The model under review builds one solid part; all positions refer to its coordinate system, in mm. Face numbers are marked on the shaded views. A direction names the side the tool comes from. Give positions to 0.01 mm unless a question says otherwise; leave off trailing zeros. Order: outer loops, then holes, each group sorted by start corner. A loop starts at its lowest first (then second) coordinate and runs counter-clockwise, first axis right, second up. Notation, with made-up numbers: (-13.5, 21.5) - (3.5, 21.5) arc R22 cw to (3.5, 55.5) - close; hole circle Ø9 at (7.25, 76). An arc over 180 degrees is marked (long way). Answer as CSV lines item,"result". Start each with the question number.
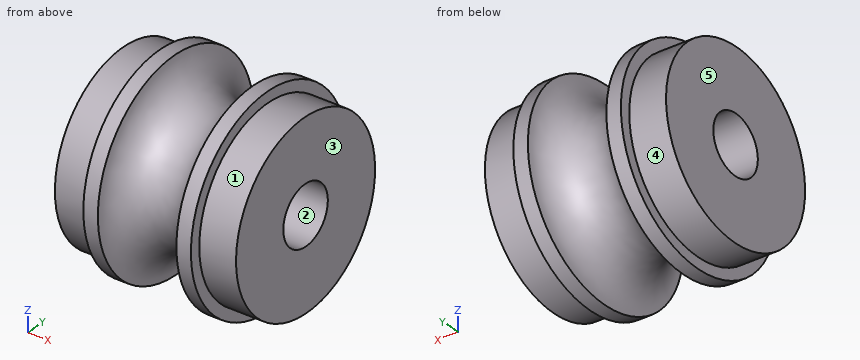
from build123d import *

# Parameters (mm, degrees)
SKETCH1_W           = 1.27
SKETCH1_H           = 8.89
SKETCH2_R           = 7.9375
BOSS_EXTRUDE1_DEPTH = 3.2131
BOSS_EXTRUDE2_START = 3.2131
SKETCH3_R           = 7.9375
BOSS_EXTRUDE2_DEPTH = 3.2131
SKETCH4_R           = 2.54
CUT_EXTRUDE1_DEPTH  = 21.210628532


with BuildPart() as part:
    # Sketch1 → Revolve1 (revolve)
    with BuildSketch(Plane.XY, mode=Mode.PRIVATE) as revolve1_sk:
        with BuildLine():
            ThreePointArc((0, 8.89), (3.429, 5.461), (6.858, 8.89))
            Line((6.858, 8.89), (6.858, 0))
            Line((6.858, 0), (0, 0))
            Line((0, 0), (0, 8.89))
        make_face()
        with Locations((-0.635, 4.445)):
            Rectangle(SKETCH1_W, SKETCH1_H)
        with Locations((7.493, 4.445)):
            Rectangle(SKETCH1_W, SKETCH1_H)
    revolve(revolve1_sk.sketch.rotate(Axis((0, 0, 0), (1, 0, 0)), 90), axis=Axis((0, 0, 0), (1, 0, 0)))

    # Sketch2 → Boss-Extrude1 (add)
    with BuildSketch(Plane(origin=(8.128, 0, 0), x_dir=(0, 0, -1), z_dir=(1, 0, 0))):
        Circle(SKETCH2_R)
    extrude(amount=BOSS_EXTRUDE1_DEPTH)

    # Sketch3 → Boss-Extrude2 (add)
    with BuildSketch(Plane.ZY.offset(1.27).offset(BOSS_EXTRUDE2_START)):
        with Locations(Location((0, 0, 0), (0, 0, 180))):
            Circle(SKETCH3_R)
    extrude(amount=-BOSS_EXTRUDE2_DEPTH)

    # Sketch4 → Cut-Extrude1 (cut, through all)
    with BuildSketch(Plane.ZY.offset(4.4831)):
        Circle(SKETCH4_R)
    extrude(amount=-CUT_EXTRUDE1_DEPTH, mode=Mode.SUBTRACT)


solid = part.part
Item 1: Take a section at D-D on x = 10. Write out the cut boundary in (y, z) (1 decimal), and give its area (3 significant figures).
Item 2: Take a section at A-A on y = 0. Write out the cut boundary in (x, z), and give its area (3 significant figures).
Item 3: Take a section at C-C on x = 7.25. Write out the cut boundary in (y, z), and give its area (3 significant figures).
Item 4: For line 1 along Z through (x, y) = (8.5, 1.75); line 2 along X through (y, z) = (6.75, 1); line 3 along X through (y, z) = (-3.75, 5.25), list the stretches that pass through material, from the lowest coordinate up.
Item 5: Clearance check with flat-ended pins moving along their axes: pin 1 (6 mm diameter, centred on x = 8, z = -5.5, fed in from -Y); pin 2 (1.5 mm diameter, centred on x = 4.5, z = -6.5, fed in from -Y). State where each tip first meets the part, or that it passes through.
Item 6: Machinability: for the marked faces 4 and 5, which of the approach directions +Z, -Z, +X, -X, +Y, -Y give a long, thin tool a straight path to every point of the face, cutting with its end or side? Answer none if there is none.
Item 7: Mouldability with a two-part tool opening along Z and no side actions: class the marked faces 1, 2 and 3 as released by +Z, released by -Z, zero draft, split by the parting line, or undercut.
Data:
1,outline,"circle Ø15.9 at (0, 0); hole circle Ø5.1 at (0, 0)"
1,area,"178 mm^2"
2,outline,"(-4.48, -7.94) - (-1.27, -7.94) - (-1.27, -8.89) - (0, -8.89) arc R3.43 cw to (6.86, -8.89) - (8.13, -8.89) - (8.13, -7.94) - (11.34, -7.94) - (11.34, -2.54) - (-4.48, -2.54) - close; (-4.48, 2.54) - (11.34, 2.54) - (11.34, 7.94) - (8.13, 7.94) - (8.13, 8.89) - (6.86, 8.89) arc R3.43 cw to (0, 8.89) - (-1.27, 8.89) - (-1.27, 7.94) - (-4.48, 7.94) - close"
2,area,"152 mm^2"
3,outline,"circle Ø17.78 at (0, 0); hole circle Ø5.08 at (0, 0)"
3,area,"228 mm^2"
4,line 1,"z = -7.74 to -1.84, 1.84 to 7.74"
4,line 2,"x = -4.48 to 0.69, 6.17 to 11.34"
4,line 3,"x = -4.48 to 1.02, 5.84 to 11.34"
5,pin 1,"stops at y = -8.53"
5,pin 2,"passes through"
6,face 4,"-X"
6,face 5,"+Z, -Z, -X, +Y, -Y"
7,face 1,"split by the parting line"
7,face 2,"undercut"
7,face 3,"zero draft"
